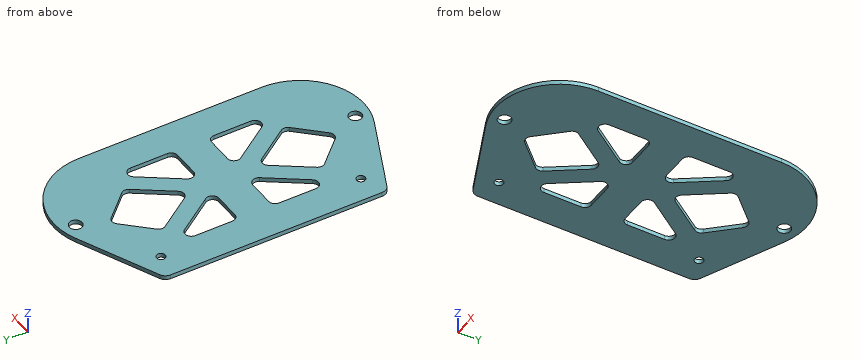
from build123d import *

# Parameters (mm, degrees)
CROQUIS3_R              = 1
CROQUIS3_R_2            = 1.500000006
CROQUIS3_R_3            = 1.000000012
CROQUIS3_R_4            = 1.5
SALIENTE_EXTRUIR1_DEPTH = 1
REDONDEO1_R             = 15
CORTAR_EXTRUIR1_DEPTH   = 1


with BuildPart() as part:
    # Croquis3 → Saliente-Extruir1 (new body)
    # profile 1 of 2: a face of its own
    with BuildSketch(Plane.XY):
        with BuildLine():
            Line((-11.943236247, 28.530474649), (-52.980665481, 28.530474649))
            Line((-52.980665481, 28.530474649), (-52.980665481, 3.561485174))
            ThreePointArc((-52.980665481, 3.561485174), (-52.660950937, 2.476754431), (-51.804024696, 1.738827882))
            Line((-51.804024696, 1.738827882), (-11.943236247, -16.267709961))
            Line((-11.943236247, -16.267709961), (-11.943236247, 28.530474649))
        make_face()
        with Locations((-47.027941845, 4.944189889)):
            Circle(CROQUIS3_R, mode=Mode.SUBTRACT)
        with Locations((-29.506723336, -4.454119513)):
            Circle(CROQUIS3_R_2, mode=Mode.SUBTRACT)
    # profile 2 of 2: a face of its own
    with BuildSketch(Plane.XY):
        with BuildLine():
            ThreePointArc((-51.804024696, 55.322121417), (-52.660950937, 54.584194868), (-52.980665481, 53.499464125))
            Line((-52.980665481, 53.499464125), (-52.980665481, 28.530474649))
            Line((-52.980665481, 28.530474649), (-11.943236247, 28.530474649))
            Line((-11.943236247, 28.530474649), (-11.943236247, 73.32865926))
            Line((-11.943236247, 73.32865926), (-51.804024696, 55.322121417))
        make_face()
        with Locations((-47.027941845, 52.116759452)):
            Circle(CROQUIS3_R_3, mode=Mode.SUBTRACT)
        with Locations((-29.506723336, 61.515068812)):
            Circle(CROQUIS3_R_4, mode=Mode.SUBTRACT)
    extrude(amount=SALIENTE_EXTRUIR1_DEPTH)

    # Redondeo1
    redondeo1_edges = [part.edges().sort_by_distance(p)[0] for p in [
        (-11.943236247, -16.267709961, 0.5),
        (-11.943236247, 73.32865926, 0.5),
    ]]
    fillet(redondeo1_edges, radius=REDONDEO1_R)

    # Croquis4 → Cortar-Extruir1 (cut)
    with BuildSketch(Plane.XY.offset(1)):
        with BuildLine():
            Line((-44.980665481, 34.030474649), (-44.980665481, 42.77886195))
            ThreePointArc((-44.980665481, 42.77886195), (-43.932223122, 44.209279965), (-42.252537885, 43.64008353))
            Line((-42.252537885, 43.64008353), (-36.117751927, 34.891696229))
            ThreePointArc((-36.117751927, 34.891696229), (-36.015121774, 33.338315841), (-37.345879522, 32.530474649))
            Line((-37.345879522, 32.530474649), (-43.480665481, 32.530474649))
            ThreePointArc((-43.480665481, 32.530474649), (-44.541325653, 32.969814478), (-44.980665481, 34.030474649))
        make_face()
        with BuildLine():
            Line((-22.671363843, 43.64008353), (-28.806149801, 34.891696229))
            ThreePointArc((-28.806149801, 34.891696229), (-28.908779954, 33.338315841), (-27.578022206, 32.530474649))
            Line((-27.578022206, 32.530474649), (-21.443236247, 32.530474649))
            ThreePointArc((-21.443236247, 32.530474649), (-20.382576076, 32.969814478), (-19.943236247, 34.030474649))
            Line((-19.943236247, 34.030474649), (-19.943236247, 42.77886195))
            ThreePointArc((-19.943236247, 42.77886195), (-20.991678606, 44.209279965), (-22.671363843, 43.64008353))
        make_face()
        with BuildLine():
            Line((-33.552014817, 54.287454199), (-39.187957869, 48.325271549))
            ThreePointArc((-39.187957869, 48.325271549), (-39.593914564, 47.404042805), (-39.326021512, 46.433632298))
            Line((-39.326021512, 46.433632298), (-33.69007846, 38.396609824))
            ThreePointArc((-33.69007846, 38.396609824), (-32.461950864, 37.757831403), (-31.233823268, 38.396609824))
            Line((-31.233823268, 38.396609824), (-25.597880217, 46.433632298))
            ThreePointArc((-25.597880217, 46.433632298), (-25.329987165, 47.404042805), (-25.735943859, 48.325271549))
            Line((-25.735943859, 48.325271549), (-31.371886911, 54.287454199))
            ThreePointArc((-31.371886911, 54.287454199), (-32.461950864, 54.757036527), (-33.552014817, 54.287454199))
        make_face()
        with BuildLine():
            Line((-31.371886911, 2.7734951), (-25.735943859, 8.73567775))
            ThreePointArc((-25.735943859, 8.73567775), (-25.329987165, 9.656906494), (-25.597880217, 10.627317001))
            Line((-25.597880217, 10.627317001), (-31.233823268, 18.664339475))
            ThreePointArc((-31.233823268, 18.664339475), (-32.461950864, 19.303117896), (-33.69007846, 18.664339475))
            Line((-33.69007846, 18.664339475), (-39.326021512, 10.627317001))
            ThreePointArc((-39.326021512, 10.627317001), (-39.593914564, 9.656906494), (-39.187957869, 8.73567775))
            Line((-39.187957869, 8.73567775), (-33.552014817, 2.7734951))
            ThreePointArc((-33.552014817, 2.7734951), (-32.461950864, 2.303912771), (-31.371886911, 2.7734951))
        make_face()
        with BuildLine():
            Line((-27.578022206, 24.530474649), (-21.443236247, 24.530474649))
            ThreePointArc((-21.443236247, 24.530474649), (-20.382576076, 24.091134821), (-19.943236247, 23.030474649))
            Line((-19.943236247, 23.030474649), (-19.943236247, 14.282087348))
            ThreePointArc((-19.943236247, 14.282087348), (-20.991678606, 12.851669334), (-22.671363843, 13.420865769))
            Line((-22.671363843, 13.420865769), (-28.806149801, 22.16925307))
            ThreePointArc((-28.806149801, 22.16925307), (-28.908779954, 23.722633457), (-27.578022206, 24.530474649))
        make_face()
        with BuildLine():
            Line((-37.345879522, 24.530474649), (-43.480665481, 24.530474649))
            ThreePointArc((-43.480665481, 24.530474649), (-44.541325653, 24.091134821), (-44.980665481, 23.030474649))
            Line((-44.980665481, 23.030474649), (-44.980665481, 14.282087348))
            ThreePointArc((-44.980665481, 14.282087348), (-43.932223122, 12.851669334), (-42.252537885, 13.420865769))
            Line((-42.252537885, 13.420865769), (-36.117751927, 22.16925307))
            ThreePointArc((-36.117751927, 22.16925307), (-36.015121774, 23.722633457), (-37.345879522, 24.530474649))
        make_face()
    extrude(amount=-CORTAR_EXTRUIR1_DEPTH, mode=Mode.SUBTRACT)


solid = part.part
Design review of the part built by this model. Coordinates are the model's own, in mm. Round coordinates to 2 decimals unless told otherwise and drop trailing zeros. Loops run counter-clockwise (first coordinate to the right, second up) from the corner with the lowest first, then second, coordinate; pieces in that order, holes last. Notation, with made-up numbers: (71, 3) - (94, 3) arc R25 ccw to (94, 40) - close; hole circle Ø3 at (73, -11.5). An arc over 180 degrees is marked (long way). One line per item, written item: value. Start each with the question number.
1) Consider section B-B on x = -30. Give the boundary of the cut face in (y, z).
2) Consider section C-C on x = -40.5. Give the boundary of the cut face in (y, z).
3) Consider section A-A on y = 37. Give the boundary of the cut face in (x, z), then the cut area to 3 significant figures.
4) To check wall thickness, follow L1, parallel to Y at x = -23.5, z = 0.35; L2, parallel to Y at x = -21.5, z = 0.25; L3, parallel to X at y = 39.5, z = 0.5. State the ranges of each line that lie inside material, in increasing order. Write a range as from..to.
5) Insertion check: pin 1 Ø2.5 at (x, y) = (-29.51, 61.52) entering from -Z; pin 2 Ø5 at (x, y) = (-29.51, -4.45) entering from +Z. Each pin has a flat end and moves straight along its axis. Give the tip position at first contact, or say it passes through.
6) Consider section D-D on z = 0.4. Give the number of separate pieces and of enclosed holes in the cut face, then the cut area to 3 significant figures.
Reported:
1. outline: (-7.72, 0) - (-5.87, 0) - (-5.87, 1) - (-7.72, 1) - close; (-3.04, 0) - (4.22, 0) - (4.22, 1) - (-3.04, 1) - close; (16.9, 0) - (40.16, 0) - (40.16, 1) - (16.9, 1) - close; (52.84, 0) - (60.1, 0) - (60.1, 1) - (52.84, 1) - close; (62.93, 0) - (64.78, 0) - (64.78, 1) - (62.93, 1) - close
2. outline: (-3.37, 0) - (15.92, 0) - (15.92, 1) - (-3.37, 1) - close; (24.53, 0) - (32.53, 0) - (32.53, 1) - (24.53, 1) - close; (41.14, 0) - (60.43, 0) - (60.43, 1) - (41.14, 1) - close
3. outline: (-52.98, 0) - (-44.98, 0) - (-44.98, 1) - (-52.98, 1) - close; (-37.6, 0) - (-27.33, 0) - (-27.33, 1) - (-37.6, 1) - close; (-19.94, 0) - (-11.94, 0) - (-11.94, 1) - (-19.94, 1) - close
3. area: 26.3 mm^2
4. L1: y = -7.63..14.6, 24.53..32.53, 42.46..64.69
4. L2: y = -7.01..12.78, 24.53..32.53, 44.28..64.07
4. L3: x = -52.98..-44.98, -39.35..-34.46, -30.46..-25.57, -19.94..-11.94
5. pin 1: passes through
5. pin 2: stops at z = 1
6. separate pieces: 1
6. enclosed holes: 10
6. area: 2,080 mm^2
